Part model, mm, in its own coordinate system. A direction names the side the tool comes from. Give positions to 0.01 mm unless a question says otherwise; leave off trailing zeros. Loops run counter-clockwise (first coordinate to the right, second up) from the corner with the lowest first, then second, coordinate; pieces in that order, holes last. Notation, with made-up numbers: (-25, 21.5) -> (7, 21.5) arc R27 cw to (7, 39.5) -> close; hole circle Ø2 at (50.5, 0). An arc over 180 degrees is marked (long way). Write item = value, one per line.
from build123d import *

# Parameters (mm, degrees)
SKETCH1_R              = 17.5
BASE_EXTRUDE_DEPTH     = 8
PROCESS_BENDS1_START   = 80
PROCESS_BENDS1_DEPTH   = 107
PROCESS_BENDS1_2_DEPTH = 107
PROCESS_BENDS1_START_2 = -196
PROCESS_BENDS1_3_DEPTH = 34.029061455


with BuildPart() as part:
    # Sketch1 → Base-Extrude (new body)
    with BuildSketch(Plane.XY):
        with BuildLine():
            Line((83, -332.5), (184, -332.5))
            ThreePointArc((184, -332.5), (186.121320344, -331.621320344), (187, -329.5))
            Line((187, -329.5), (187, -180.5))
            ThreePointArc((187, -180.5), (188.464466094, -176.964466094), (192, -175.5))
            Line((192, -175.5), (217, -175.5))
            ThreePointArc((217, -175.5), (219.121320344, -174.621320344), (220, -172.5))
            Line((220, -172.5), (220, -163.832674563))
            ThreePointArc((220, -163.832674563), (218.112603612, -156.548470658), (212.925383131, -151.097357439))
            Line((212.925383131, -151.097357439), (147.880138289, -110.618704164))
            ThreePointArc((147.880138289, -110.618704164), (140.259841851, -105.372411008), (133.157005065, -99.444323689))
            Line((133.157005065, -99.444323689), (39.541737093, -13.661735283))
            ThreePointArc((39.541737093, -13.661735283), (36.185639292, -8.978306226), (35, -3.339852568))
            Line((35, -3.339852568), (35, 27.261127274))
            ThreePointArc((35, 27.261127274), (34.942355841, 27.84639824), (34.771638598, 28.409177571))
            Line((34.771638598, 28.409177571), (25.767102684, 50.148050297))
            ThreePointArc((25.767102684, 50.148050297), (24.662174785, 51.494408837), (22.995464086, 52))
            Line((22.995464086, 52), (-37, 52))
            ThreePointArc((-37, 52), (-39.121320344, 51.121320344), (-40, 49))
            Line((-40, 49), (-40, 0))
            ThreePointArc((-40, 0), (-38.490793042, -10.883880327), (-34.077057451, -20.946459259))
            Line((-34.077057451, -20.946459259), (-4.080577734, -69.746676518))
            ThreePointArc((-4.080577734, -69.746676518), (1.377930614, -74.984191681), (8.69831881, -76.891754296))
            Line((8.69831881, -76.891754296), (20.352408817, -76.891754296))
            ThreePointArc((20.352408817, -76.891754296), (37.019515808, -81.947665927), (48.068794793, -95.411251325))
            Line((48.068794793, -95.411251325), (76.193976626, -163.311446751))
            ThreePointArc((76.193976626, -163.311446751), (79.03926402, -172.691102268), (80, -182.445618369))
            Line((80, -182.445618369), (80, -329.5))
            ThreePointArc((80, -329.5), (80.878679656, -331.621320344), (83, -332.5))
        make_face()
        Circle(SKETCH1_R, mode=Mode.SUBTRACT)
        with BuildLine():
            ThreePointArc((7.863280204, -55.950145884), (14.146470229, -54.700341681), (20.247789149, -52.747294097))
            ThreePointArc((20.247789149, -52.747294097), (27.999479406, -56.198568959), (24.548204544, -63.950259215))
            ThreePointArc((24.548204544, -63.950259215), (17.151030278, -66.318113366), (9.533357416, -67.833362709))
            ThreePointArc((9.533357416, -67.833362709), (2.756710398, -62.726792902), (7.863280204, -55.950145884))
        make_face(mode=Mode.SUBTRACT)
    extrude(amount=-BASE_EXTRUDE_DEPTH)

    # Process-Bends1: read off the stored shape, not the designer's step
    # Process-Bends1 outline → Process-Bends1 (cut)
    with BuildSketch(Plane.YZ.offset(PROCESS_BENDS1_START)):
        with BuildLine():
            Line((-332.5, -8), (-216.824957909, -8))
            ThreePointArc((-216.824957909, -8), (-207.812045211, -2.077037206), (-197.229039967, 0))
            Line((-197.229039967, 0), (-332.5, 0))
            Line((-332.5, 0), (-332.5, -8))
        make_face()
    extrude(amount=PROCESS_BENDS1_DEPTH, mode=Mode.SUBTRACT)

    # Process-Bends1 2 outline → Process-Bends1 2 (add)
    with BuildSketch(Plane.YZ.offset(PROCESS_BENDS1_START)):
        with BuildLine():
            Line((-268.556535875, -114.70866427), (-261.306073579, -118.089610364))
            Line((-261.306073579, -118.089610364), (-215.355195707, -19.547634765))
            ThreePointArc((-215.355195707, -19.547634765), (-207.975032134, -11.132171084), (-197.229039967, -8))
            Line((-197.229039967, -8), (-216.824957909, -8))
            ThreePointArc((-216.824957909, -8), (-220.083053817, -11.823039502), (-222.605658004, -16.166688671))
            Line((-222.605658004, -16.166688671), (-268.556535875, -114.70866427))
        make_face()
    extrude(amount=PROCESS_BENDS1_2_DEPTH)

    # Process-Bends1 3 outline → Process-Bends1 3 (cut)
    with BuildSketch(Plane(origin=(0, 0, 0), x_dir=(1, 0, 0), z_dir=(0, 0.9063077870366512, -0.42261826174069705)).offset(PROCESS_BENDS1_START_2)):
        with BuildLine():
            Line((187, 217.458252039), (184, 217.458252039))
            ThreePointArc((184, 217.458252039), (186.121320344, 216.579572383), (187, 214.458252039))
            Line((187, 214.458252039), (187, 217.458252039))
        make_face()
        with BuildLine():
            ThreePointArc((80, 214.458252039), (80.878679656, 216.579572383), (83, 217.458252039))
            Line((83, 217.458252039), (80, 217.458252039))
            Line((80, 217.458252039), (80, 214.458252039))
        make_face()
    extrude(amount=PROCESS_BENDS1_3_DEPTH, mode=Mode.SUBTRACT)


solid = part.part
1) Which spindle directions (+Z, -Z, +X, -X, +Y, -Y) get a long thin tool onto all of the face, cutting with end or side? Do faces 4 (the face through (35, 12, -4)), 5 (the face through (187, -231, -49)), 6 (the face through (14, -76.892, -4)). Say none if no direction does.
Resolved:
face_4 = +Z, -Z, +X, +Y
face_5 = +Z, -Z, +X, -Y
face_6 = +Z, -Z, -X, -Y
2) Drill centre lines: line 1 along Y through (x, z) = (0, -4.25); line 2 along Z through (x, y) = (142, -165.5); line 3 along Z through (x, y) = (178.5, -246). Where is each one in solid material? Low to high. Write a range as [from, to].
Resolved:
line_1 = [-74.11, -17.5], [17.5, 52]
line_2 = [-8, 0]
line_3 = [-85.27, -66.34]
3) Pull direction Y, two halves, no side cores. Call faces 1 (the face through (180.858, -131.141, -3.944)), 2 (the face through (204, -175.5, -4)), 3 (the face through (14.06, -54.723, -3.944)): pulls with the +Y half, pulls with the -Y half, needs draft (parallel to the pull), parting line crosses it, or undercut.
Resolved:
face_1 = pulls with the +Y half
face_2 = pulls with the -Y half
face_3 = undercut
4) Slice it at A-A, the plane x = 167. List the corners of the cut face in (y, z), and give its area (3 significant figures).
Resolved:
outline = (-268.56, -114.71) -> (-261.31, -118.09) -> (-215.36, -19.55) arc R20 cw to (-197.23, -8) -> (-122.52, -8) -> (-122.52, 0) -> (-197.23, 0) arc R28 ccw to (-222.61, -16.17) -> close
area = 1,690 mm²
5) Slice it at B-B, the plane z = -74.5. List the corners of the cut face in (x, y), and give its area (3 significant figures).
Resolved:
outline = (80, -249.81) -> (187, -249.81) -> (187, -240.98) -> (80, -240.98) -> close
area = 944 mm²
6) Drop flat-ended pins along their axis: P1, Ø1.5, axis at x = 106, y = -75.5, coming from the -Z side; P2, Ø2, axis at x = 113, z = -15.5, coming from the +Y side; P3, Ø6.5, axis at y = 5.5, z = -4, coming from the +X side. Give the stop position or say it passes through.
Resolved:
P1 = -8
P2 = -211.99
P3 = 35
7) Slice it at C-C, the plane y = -86. List the corners of the cut face in (x, z).
Resolved:
outline = (41.88, -8) -> (118.49, -8) -> (118.49, 0) -> (41.88, 0) -> close
8) Slice it at D-D, the plane x = 126.5. List the corners of the cut face in (y, z).
Resolved:
outline = (-268.56, -114.71) -> (-261.31, -118.09) -> (-215.36, -19.55) arc R20 cw to (-197.23, -8) -> (-93.34, -8) -> (-93.34, 0) -> (-197.23, 0) arc R28 ccw to (-222.61, -16.17) -> close
